Geometry: see drawing. Coordinates: mm, zero at the bounding-box minimum. A direction names the side the tool comes from. Round coordinates to 2 decimals unless told otherwise and drop trailing zeros. Loops run counter-clockwise (first coordinate to the right, second up) from the corner with the lowest first, then second, coordinate; pieces in that order, holes last.
(1) Section C-C, the plane x = 24. Return the cut outline in (y, z), plus the area to 3 significant figures.
(2) Set-up query: the marked faces 4, 5 and 6. Return all of +Z, -Z, +X, -X, +Y, -Y with unobstructed straight access to the full face (end or side cutting, diameter ignored); none if empty.
(3) Section A-A, the plane y = 6.75. Return the cut outline in (x, z), plus the area to 3 significant figures.
(4) Section B-B, the plane z = 70. Return the cut outline in (x, y).
(5) Material intervals for probe 1 along X at (y, z) = (1.05, 30); probe 2 along X at (y, z) = (7, 45); probe 3 along Z at (x, y) = (13, 5.5), sorted ascending.
(6) Mould query, pull axis Z, two halves, no side actions, for the marked faces 1, 2 and 3. Classes: pulls with the +Z half, pulls with the -Z half, needs draft (parallel to the pull), parting line crosses it, or undercut.
(7) First-contact query: pin 1 Ø8 at (y, z) = (7.5, 9.5) entering from -X; pin 2 Ø5.5 at (x, y) = (22, 20) entering from -Z; pin 3 Ø1.5 at (x, y) = (13, 14) entering from -Z; pin 4 Ø9 at (x, z) = (9.5, 60) entering from +Y. Flat tips, straight axial feed; report the tip coordinate or a pass-through.
(8) Section D-D, the plane z = 56. Return the cut outline in (x, y), plus the area to 3 significant figures.
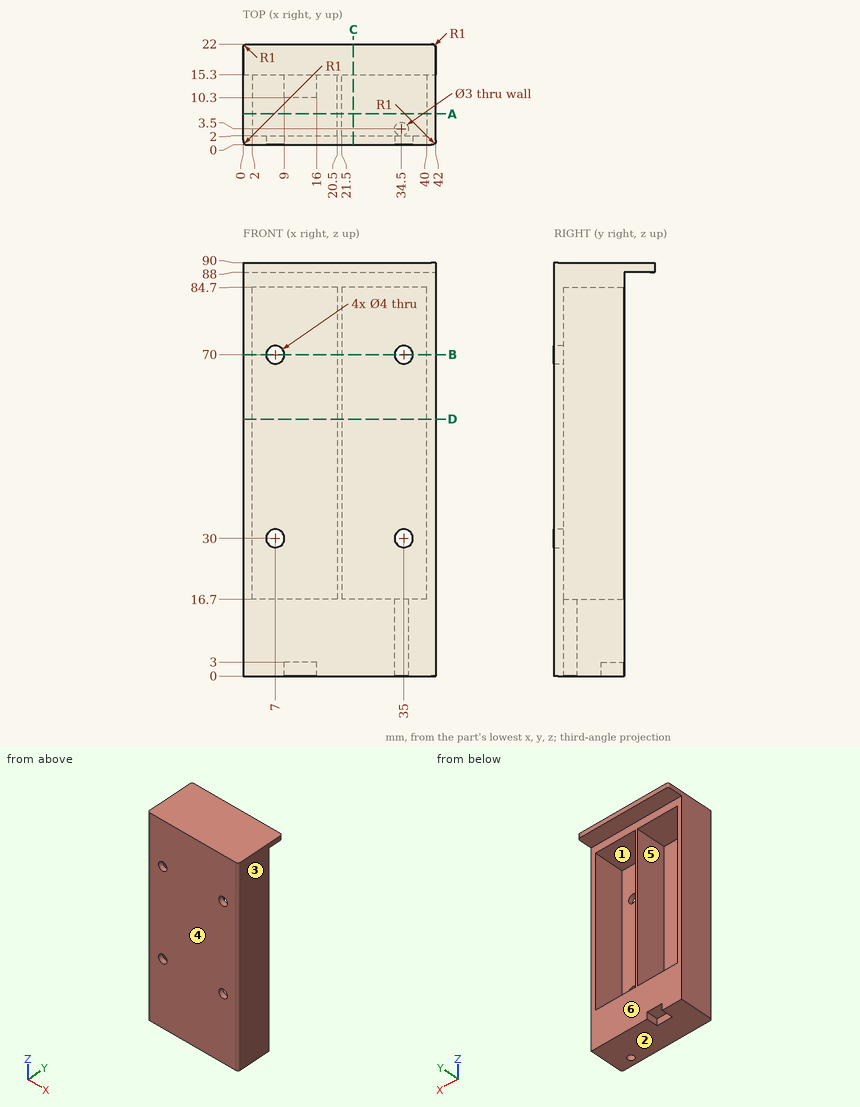
Output values:
1. outline: (0, 0) - (15.3, 0) - (15.3, 16.7) - (2, 16.7) - (2, 84.7) - (15.3, 84.7) - (15.3, 88) - (22, 88) - (22, 90) - (0, 90) - close
1. area: 486 mm2
2. face 4: +Z, -Z, +X, -X, -Y
2. face 5: +Y
2. face 6: -Z, +X, -X, +Y
3. outline: (0, 0) - (42, 0) - (42, 90) - (0, 90) - close; hole (2, 16.7) - (20.5, 16.7) - (20.5, 84.7) - (2, 84.7) - close; hole (21.5, 16.7) - (40, 16.7) - (40, 84.7) - (21.5, 84.7) - close
3. area: 1,260 mm2
4. outline: (0, 1) arc R1 ccw to (1, 0) - (5, 0) - (5, 2) - (2, 2) - (2, 15.3) - (0, 15.3) - close; (9, 0) - (33, 0) - (33, 2) - (21.5, 2) - (21.5, 15.3) - (20.5, 15.3) - (20.5, 2) - (9, 2) - close; (37, 0) - (41, 0) arc R1 ccw to (42, 1) - (42, 15.3) - (40, 15.3) - (40, 2) - (37, 2) - close
5. probe 1: x = 0 to 5, 9 to 33, 37 to 42
5. probe 2: x = 0 to 2, 20.5 to 21.5, 40 to 42
5. probe 3: z = 0 to 16.7, 84.7 to 90
6. face 1: undercut
6. face 2: pulls with the -Z half
6. face 3: needs draft
7. pin 1: stops at x = 0
7. pin 2: stops at z = 88
7. pin 3: stops at z = 3
7. pin 4: stops at y = 2
8. outline: (0, 1) arc R1 ccw to (1, 0) - (41, 0) arc R1 ccw to (42, 1) - (42, 15.3) - (40, 15.3) - (40, 2) - (21.5, 2) - (21.5, 15.3) - (20.5, 15.3) - (20.5, 2) - (2, 2) - (2, 15.3) - (0, 15.3) - close
8. area: 150 mm2
